Verification items for the finished model (mm, model axes). Face numbers are marked on the shaded views. A direction names the side the tool comes from. Coordinates: 2 decimals unless noted, no trailing zeros. Order: outer loops, then holes, each group sorted by start corner. A loop starts at its lowest first (then second) coordinate and runs counter-clockwise, first axis right, second up. Notation, with made-up numbers: (-29.75, 74.25) -> (-1.75, 74.25) arc R21 cw to (-1.75, 110.25) -> close; hole circle Ø3 at (59.25, 19). An arc over 180 degrees is marked (long way). Write item = value, one per line. Start each with the question number.
1. Cross-section at B-B on z = 74.8. Record the cut outline in (x, y), plus the area to 3 significant figures.
2. Release check for a two-part mould opening along Z. For the marked faces 1, 2 and 3 record: +Z half, -Z half, draft (parallel to the pull), parting line (faces both ways), or undercut.
3. Set-up check for the marked faces 4 and 5: record each of +Z, -Z, +X, -X, +Y, -Y from which the full face is reachable in a straight line by a thin tool's end or side.
4. Cross-section at A-A on x = 2. Record the cut outline in (y, z), plus the area to 3 significant figures.
5. Cross-section at C-C on y = 45. Record the cut outline in (x, z), plus the area to 3 significant figures.
6. Thickness scan on line 1 along X through (y, z) = (58.75, 74.8); line 2 along Y through (x, z) = (-4.5, 11.5); line 3 along Z through (x, y) = (25, 39). Record the ranges inside material, lowest first. Write a range as from..to.
7. Go/stop test with flat-tipped pins: P1, Ø1, axis at x = -2.5, y = 58.5, coming from the +Z side; P2, Ø4, axis at x = 23, z = 7.8, coming from the +Y side; P3, Ø5, axis at x = 15.5, y = -3, coming from the +Z side; P4, Ø1, axis at x = 20.5, z = 83, coming from the -Y side. Record where each tip stops, or that it passes through.
8. Cross-section at D-D on y = 21. Record the cut outline in (x, z).
from build123d import *

# Parameters (mm, degrees)
SKETCH_1_W                       = 35
SKETCH_1_H                       = 68
SKETCH_1_R                       = 2
SKETCH_1_W_2                     = 21
SKETCH_1_H_2                     = 42
SM_BASE_FLANGE_1_DEPTH           = 1.2
SM_EDGE_FLANGE_1_STRIP_W         = 6.2732
SM_EDGE_FLANGE_1_STRIP_H         = 1.2
SM_EDGE_FLANGE_1_STRIP_CUT_DEPTH = 35
SM_EDGE_FLANGE_1_DEPTH           = 35
SM_EDGE_FLANGE_1_FLAT_DEPTH      = 1.2
SM_EDGE_FLANGE_2_STRIP_W         = 6.2732
SM_EDGE_FLANGE_2_STRIP_H         = 1.2
SM_EDGE_FLANGE_2_STRIP_CUT_DEPTH = 24
SM_EDGE_FLANGE_2_DEPTH           = 24
CUT_EXTRUDE_1_REACH              = 109.191
SKETCH_12_R                      = 2.25
CUT_EXTRUDE_2_REACH              = 113.492
SKETCH_13_R                      = 2.25


# Sheet-metal steps are written as plain solids
with BuildPart() as part:
    # Sketch 1 → Базовая кромка1 (new body)
    with BuildSketch(Plane.XY):
        with Locations((10.5, 25)):
            Rectangle(SKETCH_1_W, SKETCH_1_H)
        with Locations((5.5, 45)):
            Circle(SKETCH_1_R, mode=Mode.SUBTRACT)
        with Locations((15.5, 45)):
            Circle(SKETCH_1_R, mode=Mode.SUBTRACT)
        with Locations((5.5, -3)):
            Circle(SKETCH_1_R, mode=Mode.SUBTRACT)
        with Locations((15.5, -3)):
            Circle(SKETCH_1_R, mode=Mode.SUBTRACT)
        with Locations((10.5, 21)):
            Rectangle(SKETCH_1_W_2, SKETCH_1_H_2, mode=Mode.SUBTRACT)
    extrude(amount=-SM_BASE_FLANGE_1_DEPTH)

    # Ребро-кромка1 strip (across the edge) → Ребро-кромка1 strip cut (cut)
    with BuildSketch(Plane(origin=(28, 59, 0), x_dir=(0, -1, 0), z_dir=(-1, 0, 0))):
        with Locations((-1.2, -0.6)):
            Rectangle(SM_EDGE_FLANGE_1_STRIP_W, SM_EDGE_FLANGE_1_STRIP_H)
    extrude(amount=SM_EDGE_FLANGE_1_STRIP_CUT_DEPTH, mode=Mode.SUBTRACT)

    # Ребро-кромка1 bend section (across the edge) → Ребро-кромка1 (add)
    with BuildSketch(Plane(origin=(28, 59, 0), x_dir=(0, -1, 0), z_dir=(-1, 0, 0))):
        with BuildLine():
            Line((0, 0.7366), (1.2, 0.7366))
            ThreePointArc((1.2, 0.7366), (1.415745145, 0.215745145), (1.9366, 0))
            Line((1.9366, 0), (1.9366, -1.2))
            ThreePointArc((1.9366, -1.2), (0.567217008, -0.632782992), (0, 0.7366))
        make_face()
    extrude(amount=SM_EDGE_FLANGE_1_DEPTH)

    # Ребро-кромка1 profile (on flange) → Ребро-кромка1 flat (add)
    with BuildSketch(Plane(origin=(0, 59, 0), x_dir=(-1, 0, 0), z_dir=(0, 1, 0))):
        Polygon((-28, 83.8), (-28, 0.7366), (7, 0.7366), (7, 15), (-4, 15), (-4, 83.8), align=None)
    extrude(amount=-SM_EDGE_FLANGE_1_FLAT_DEPTH)

    # Ребро-кромка2 strip (across the edge) → Ребро-кромка2 strip cut (cut)
    with BuildSketch(Plane(origin=(28, 57.8, 83.8), x_dir=(0, 0, -1), z_dir=(-1, 0, 0))):
        with Locations((-1.2, -0.6)):
            Rectangle(SM_EDGE_FLANGE_2_STRIP_W, SM_EDGE_FLANGE_2_STRIP_H)
    extrude(amount=SM_EDGE_FLANGE_2_STRIP_CUT_DEPTH, mode=Mode.SUBTRACT)

    # Ребро-кромка2 section (across the edge) → Ребро-кромка2 (add)
    with BuildSketch(Plane(origin=(28, 57.8, 83.8), x_dir=(0, 0, -1), z_dir=(-1, 0, 0))):
        with BuildLine():
            Line((0, 0.7366), (0, 33))
            Line((0, 33), (1.2, 33))
            Line((1.2, 33), (1.2, 0.7366))
            ThreePointArc((1.2, 0.7366), (1.415745145, 0.215745145), (1.9366, 0))
            Line((1.9366, 0), (1.9366, -1.2))
            ThreePointArc((1.9366, -1.2), (0.567217008, -0.632782992), (0, 0.7366))
        make_face()
    extrude(amount=SM_EDGE_FLANGE_2_DEPTH)

    # Эскиз12 → Вырез-Вытянуть1 (cut, up to next)
    with BuildSketch(Plane.XY.offset(83.8), mode=Mode.PRIVATE) as cut_extrude_1_sk1:
        with Locations((10.419999997, 31.03)):
            Circle(SKETCH_12_R)
    cut_extrude_1_tool1 = extrude(cut_extrude_1_sk1.sketch, amount=-CUT_EXTRUDE_1_REACH, mode=Mode.PRIVATE) & part.part
    add(cut_extrude_1_tool1.solids().sort_by_distance((10.42, 31.03, 83.8))[0], mode=Mode.SUBTRACT)

    # Эскиз13 → Вырез-Вытянуть2 (cut, up to next)
    with BuildSketch(Plane(origin=(0, 59, 0), x_dir=(1, 0, 0), z_dir=(0, 1, 0)), mode=Mode.PRIVATE) as cut_extrude_2_sk1:
        with Locations(Location((23, -7.8, 0), (0, 0, 270))):
            Circle(SKETCH_13_R)
    cut_extrude_2_tool1 = extrude(cut_extrude_2_sk1.sketch, amount=-CUT_EXTRUDE_2_REACH, mode=Mode.PRIVATE) & part.part
    # Эскиз13 → Вырез-Вытянуть2 (cut, up to next)
    with BuildSketch(Plane(origin=(0, 59, 0), x_dir=(1, 0, 0), z_dir=(0, 1, 0)), mode=Mode.PRIVATE) as cut_extrude_2_sk2:
        with Locations(Location((-2, -7.8, 0), (0, 0, 270))):
            Circle(SKETCH_13_R)
    cut_extrude_2_tool2 = extrude(cut_extrude_2_sk2.sketch, amount=-CUT_EXTRUDE_2_REACH, mode=Mode.PRIVATE) & part.part
    # Эскиз13 → Вырез-Вытянуть2 (cut, up to next)
    with BuildSketch(Plane(origin=(0, 59, 0), x_dir=(1, 0, 0), z_dir=(0, 1, 0)), mode=Mode.PRIVATE) as cut_extrude_2_sk3:
        with Locations(Location((9, -74.8, 0), (0, 0, 270))):
            Circle(SKETCH_13_R)
    cut_extrude_2_tool3 = extrude(cut_extrude_2_sk3.sketch, amount=-CUT_EXTRUDE_2_REACH, mode=Mode.PRIVATE) & part.part
    # Эскиз13 → Вырез-Вытянуть2 (cut, up to next)
    with BuildSketch(Plane(origin=(0, 59, 0), x_dir=(1, 0, 0), z_dir=(0, 1, 0)), mode=Mode.PRIVATE) as cut_extrude_2_sk4:
        with Locations(Location((23, -74.8, 0), (0, 0, 270))):
            Circle(SKETCH_13_R)
    cut_extrude_2_tool4 = extrude(cut_extrude_2_sk4.sketch, amount=-CUT_EXTRUDE_2_REACH, mode=Mode.PRIVATE) & part.part
    add(cut_extrude_2_tool1.solids().sort_by_distance((23, 59, 7.8))[0], mode=Mode.SUBTRACT)
    add(cut_extrude_2_tool2.solids().sort_by_distance((-2, 59, 7.8))[0], mode=Mode.SUBTRACT)
    add(cut_extrude_2_tool3.solids().sort_by_distance((9, 59, 74.8))[0], mode=Mode.SUBTRACT)
    add(cut_extrude_2_tool4.solids().sort_by_distance((23, 59, 74.8))[0], mode=Mode.SUBTRACT)


solid = part.part
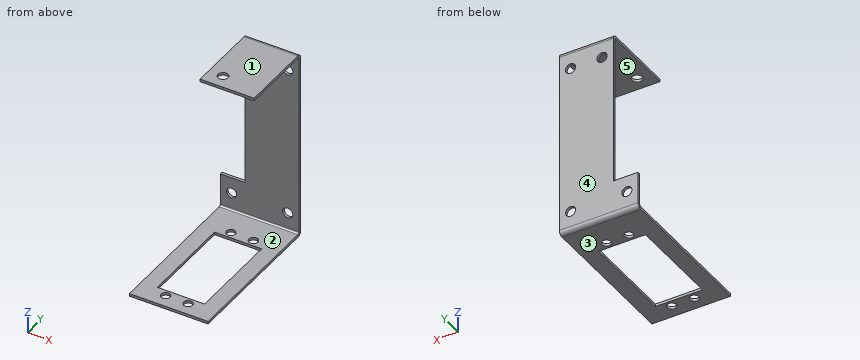
Worked out:
q1.outline = (4, 57.8) -> (6.75, 57.8) -> (6.75, 59) -> (4, 59) -> close; (11.25, 57.8) -> (20.75, 57.8) -> (20.75, 59) -> (11.25, 59) -> close; (25.25, 57.8) -> (28, 57.8) -> (28, 59) -> (25.25, 59) -> close
q1.area = 18.0 mm²
q2.face_1 = +Z half
q2.face_2 = undercut
q2.face_3 = -Z half
q3.face_4 = +Z, -Z, +X, -X, +Y
q3.face_5 = +X, -X, -Y
q4.outline = (-9, -1.2) -> (0, -1.2) -> (0, 0) -> (-9, 0) -> close; (42, -1.2) -> (57.06, -1.2) arc R1.94 ccw to (59, 0.74) -> (59, 15) -> (57.8, 15) -> (57.8, 0.74) arc R0.74 cw to (57.06, 0) -> (42, 0) -> close
q4.area = 48.5 mm²
q5.outline = (-7, -1.2) -> (3.5, -1.2) -> (3.5, 0) -> (-7, 0) -> close; (4, 82.6) -> (28, 82.6) -> (28, 83.8) -> (4, 83.8) -> close; (7.5, -1.2) -> (13.5, -1.2) -> (13.5, 0) -> (7.5, 0) -> close; (17.5, -1.2) -> (28, -1.2) -> (28, 0) -> (17.5, 0) -> close
q5.area = 61.2 mm²
q6.line_1 = 4..6.75, 11.25..20.75, 25.25..28
q6.line_2 = 57.8..59
q6.line_3 = -1.2..0, 82.6..83.8
q7.P1 = 15
q7.P2 = through
q7.P3 = 0
q7.P4 = 24.8
q8.outline = (-7, -1.2) -> (0, -1.2) -> (0, 0) -> (-7, 0) -> close; (21, -1.2) -> (28, -1.2) -> (28, 0) -> (21, 0) -> close
